Read the model definition and answer for the solid it produces. Units are mm, in the model's axes. Face numbers are marked on the shaded views. A direction names the side the tool comes from. Give positions to 0.01 mm unless a question says otherwise; leave off trailing zeros. Write each loop counter-clockwise with the first axis right and the second up, starting at its lowest first coordinate (ties: lowest second). Pieces come first, ordered by that corner, then holes.
```python
from build123d import *

# Parameters (mm, degrees)
F0_W     = 60
F0_H     = 50
F0_R     = 14.1543173952
F1_DEPTH = 30
F2_W     = 20.1585159823
F2_H     = 10.1142704487
F3_DEPTH = 95
F4_W     = 20
F4_H     = 9.8414840177
F5_DEPTH = 10


with BuildPart() as f1:
    # F0 (on Front) → F1 (new body)
    with BuildSketch(Plane.XZ):
        with Locations((0, 25)):
            Rectangle(F0_W, F0_H)
        with Locations((0, 25)):
            Circle(F0_R, mode=Mode.SUBTRACT)
    extrude(amount=F1_DEPTH)

    # F2 (on face) → F3 (cut)
    with BuildSketch(Plane.YZ.offset(30)):
        with Locations((-19.9207420088, 44.9428647757)):
            Rectangle(F2_W, F2_H)
    extrude(amount=-F3_DEPTH, mode=Mode.SUBTRACT)

    # F4 (on face) → F5 (cut)
    with BuildSketch(Plane.XY.offset(50)):
        with Locations((0, -4.9207420088)):
            Rectangle(F4_W, F4_H)
    extrude(amount=-F5_DEPTH, mode=Mode.SUBTRACT)


solid = f1.part
```
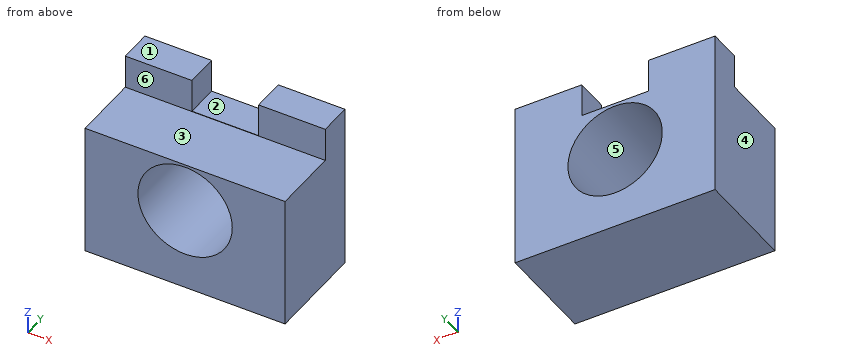
Item 1: Determine the mould class of the marked faces 4, 5 and 6 for opening direction X: pulls with the +X half, pulls with the -X half, needs draft (parallel to the pull), parting line crosses it, or undercut.
Result set:
face 4: pulls with the -X half
face 5: undercut
face 6: needs draft
Item 2: Section D-D (x = -16) is taken. Write down the section's boundary in (y, z).
Result set:
outline: (-30, 0) - (0, 0) - (0, 50) - (-9.84, 50) - (-9.84, 39.89) - (-30, 39.89) - close
Item 3: Which of the six approach directions +Z, -Z, +X, -X, +Y, -Y give full straight-line access (tool end or side, diameter ignored) to the marked faces 1, 2 and 3?
Result set:
face 1: +Z, +X, -X, +Y, -Y
face 2: +Z, +Y, -Y
face 3: +Z, +X, -X, -Y
Item 4: Section A-A (z = 25) is taken. Write down the section's boundary in (x, y).
Result set:
outline: (-30, -30) - (-14.15, -30) - (-14.15, 0) - (-30, 0) - close; (14.15, -30) - (30, -30) - (30, 0) - (14.15, 0) - close
Item 5: Each of these flat-tipped pins is pushed along its axis until it touches: pin 1 Ø5 at (x, y) = (-2.5, -5.5) entering from +Z; pin 2 Ø10 at (x, z) = (-0.5, 30.5) entering from +Y; pin 3 Ø10 at (x, y) = (-12.5, -19.5) entering from +Z. Where does it stop, or does it pass through?
Result set:
pin 1: stops at z = 40
pin 2: passes through
pin 3: stops at z = 39.89
Item 6: Section C-C (y = -8) is taken. Write down the section's boundary in (x, z), and give its area (3 significant figures).
Result set:
outline: (-30, 0) - (30, 0) - (30, 50) - (10, 50) - (10, 40) - (-10, 40) - (-10, 50) - (-30, 50) - close; hole circle Ø28.31 at (0, 25)
area: 2,170 mm2
Item 7: Find the intervals of material crossed by line 1 along Z through (x, y) = (0, -14.75); line 2 along X through (y, z) = (-6, 44); line 3 along Z through (x, y) = (20.5, -24), in increasing order.
Result set:
line 1: z = 0 to 10.85, 39.15 to 39.89
line 2: x = -30 to -10, 10 to 30
line 3: z = 0 to 39.89
Item 8: Section B-B (x = 0) is taken. Write down the section's boundary in (y, z).
Result set:
outline: (-30, 0) - (0, 0) - (0, 10.85) - (-30, 10.85) - close; (-30, 39.15) - (0, 39.15) - (0, 40) - (-9.84, 40) - (-9.84, 39.89) - (-30, 39.89) - close
